Build history of the part. All positions in model axes, mm. A direction names the side the tool comes from. Give positions to 0.01 mm unless a question says otherwise; leave off trailing zeros. Loops run counter-clockwise (first coordinate to the right, second up) from the corner with the lowest first, then second, coordinate; pieces in that order, holes last. Notation, with made-up numbers: M -22.75,77.5 L -12.75,77.5 A29 cw -12.75,105.5 Z; hole C 71,-2.75 d6. An arc over 180 degrees is marked long. Answer in a Markdown table with one row per item. Add a question column.
```python
from build123d import *

# Parameters (mm, degrees)
BOSS_EXTRU_1_DEPTH = 2
BOSS_EXTRU_2_DEPTH = 1
CONG_1_R           = 0.25


with BuildPart() as part:
    # Esquisse1 → Boss.-Extru.1 (new body)
    with BuildSketch(Plane.XY):
        with BuildLine():
            Line((-3, 1.75), (3, 1.75))
            ThreePointArc((3, 1.75), (4.75, 0), (3, -1.75))
            Line((3, -1.75), (-3, -1.75))
            ThreePointArc((-3, -1.75), (-4.75, 0), (-3, 1.75))
        make_face()
    extrude(amount=BOSS_EXTRU_1_DEPTH)

    # Esquisse3 → Boss.-Extru.2 (add)
    with BuildSketch(Plane.XY):
        with BuildLine():
            Line((-3, 2.25), (3, 2.25))
            ThreePointArc((3, 2.25), (5.25, 0), (3, -2.25))
            Line((3, -2.25), (-3, -2.25))
            ThreePointArc((-3, -2.25), (-5.25, 0), (-3, 2.25))
        make_face()
    extrude(amount=-BOSS_EXTRU_2_DEPTH)

    # Congé1
    cong_1_edges = [part.edges().sort_by_distance(p)[0] for p in [
        (4.75, 0, 2),
        (0, 1.75, 2),
        (-4.75, 0, 2),
        (0, -1.75, 2),
    ]]
    fillet(cong_1_edges, radius=CONG_1_R)


solid = part.part
```
(1) Pin check, flat tips, straight feed: pin 1 (1 mm diameter, centred on y = -1, z = 0, fed in from +X); pin 2 (1 mm diameter, centred on x = -1.5, y = -2, fed in from +Z); pin 3 (1 mm diameter, centred on y = -0.5, z = 1, fed in from -X); pin 4 (0.5 mm diameter, centred on x = -0.5, z = 0.5, fed in from -Y). Stop position of each tip, or through.
(2) Tool access for faces 1 (the flat face through (0, -1.75, 1)), 2 (the flat face through (0, 1.75, 1)), 3 (the cylindrical face through (4.75, 0.04, 0.86)), 4 (the flat face through (0, -2, 0)): list every direction of +Z, -Z, +X, -X, +Y, -Y with a clear straight run to the whole face (end or side of a thin tool).
(3) Slice it at A-A, the plane y = 0. Give the cut face in (x, z), then the cut area to 3 significant figures.
(4) Slice it at D-D, the plane z = 0.75. Give the cut face in (x, y), then the cut area to 3 significant figures.
(5) Slice it at B-B, the plane x = -2. Give the cut face in (y, z), then the cut area to 3 significant figures.
(6) Wall check: line 1 (Y direction, x = -1.75, z = 1.75); line 2 (X direction, y = -0.05, z = 1.3); line 3 (Z direction, x = -4.5, y = -1.6). Give the ranges that are in metal, low to high.
(7) Slice it at C-C, the plane z = -0.1. Give the cut face in (x, y).
Solution:
| question | item | result |
|---|---|---|
| 1 | pin 1 | x = 5.19 |
| 1 | pin 2 | z = 2 |
| 1 | pin 3 | x = -4.75 |
| 1 | pin 4 | y = -1.75 |
| 2 | face 1 | +Z, +X, -X, -Y |
| 2 | face 2 | +Z, +X, -X, +Y |
| 2 | face 3 | +Z, +X |
| 2 | face 4 | +Z |
| 3 | outline | M -5.25,-1 L 5.25,-1 L 5.25,0 L 4.75,0 L 4.75,1.75 A0.25 ccw 4.5,2 L -4.5,2 A0.25 ccw -4.75,1.75 L -4.75,0 L -5.25,0 Z |
| 3 | area | 29.5 mm^2 |
| 4 | outline | M -3,-1.75 L 3,-1.75 A1.75 ccw 3,1.75 L -3,1.75 A1.75 ccw Z |
| 4 | area | 30.6 mm^2 |
| 5 | outline | M -2.25,-1 L 2.25,-1 L 2.25,0 L 1.75,0 L 1.75,1.75 A0.25 ccw 1.5,2 L -1.5,2 A0.25 ccw -1.75,1.75 L -1.75,0 L -2.25,0 Z |
| 5 | area | 11.5 mm^2 |
| 6 | line 1 | -1.75 to 1.75 |
| 6 | line 2 | -4.75 to 4.75 |
| 6 | line 3 | -1 to 0 |
| 7 | outline | M -3,-2.25 L 3,-2.25 A2.25 ccw 3,2.25 L -3,2.25 A2.25 ccw Z |
